Build history of the part. All positions in model axes, mm. Face numbers are marked on the shaded views. A direction names the side the tool comes from. Give positions to 0.01 mm unless a question says otherwise; leave off trailing zeros. Order: outer loops, then holes, each group sorted by start corner. A loop starts at its lowest first (then second) coordinate and runs counter-clockwise, first axis right, second up. Notation, with made-up numbers: (-19.75, -6) -> (-13.75, -6) arc R21 cw to (-13.75, 1) -> close; hole circle Ø1 at (88, 80.5). An arc over 180 degrees is marked (long way). Use a Markdown table: item, result. Add a question column.
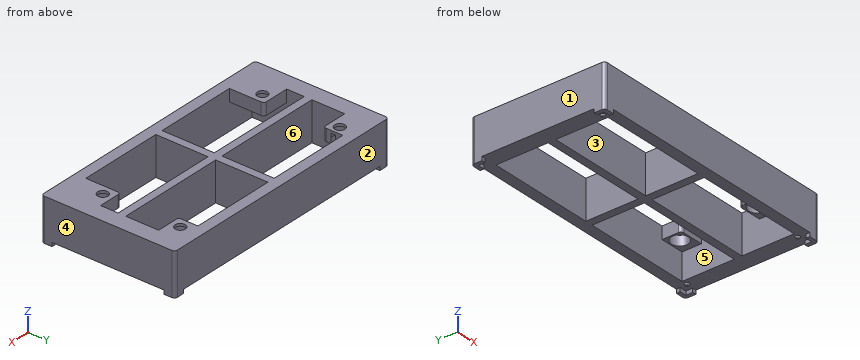
```python
from build123d import *

# Parameters (mm, degrees)
SKETCH1_W                                        = 170.1
SKETCH1_H                                        = 87.55
SKETCH1_W_2                                      = 148.1
SKETCH1_H_2                                      = 73.55
SKETCH1_W_3                                      = 71.55
SKETCH1_H_3                                      = 5
SKETCH1_W_4                                      = 5
SKETCH1_H_4                                      = 34.275
BOSS_EXTRUDE1_DEPTH                              = 25.4
SKETCH2_W                                        = 2.5
SKETCH2_H                                        = 4.5
SKETCH2_W_2                                      = 4.501529918
SKETCH2_H_2                                      = 2.5
SKETCH2_W_3                                      = 4.5
BOSS_EXTRUDE2_DEPTH                              = 2.5
SKETCH3_R                                        = 1.5
BOSS_EXTRUDE3_DEPTH                              = 1
BOSS_EXTRUDE4_DEPTH                              = 8
CBORE_FOR_1_4_SOCKET_HEAD_CAP_SCREW1_D           = 6.7564
CBORE_FOR_1_4_SOCKET_HEAD_CAP_SCREW1_CBORE_D     = 11.1125
CBORE_FOR_1_4_SOCKET_HEAD_CAP_SCREW1_CBORE_DEPTH = 6.35
FILLET1_R                                        = 1
FILLET2_R                                        = 2


with BuildPart() as part:
    # Sketch1 → Boss-Extrude1 (new body)
    # profile 1 of 6: a face of its own
    with BuildSketch(Plane.XY):
        with Locations((-57.284342841, -127.375162174)):
            Rectangle(SKETCH1_W, SKETCH1_H)
        with Locations((-57.284342841, -127.375162174)):
            Rectangle(SKETCH1_W_2, SKETCH1_H_2, mode=Mode.SUBTRACT)
    # profile 2 of 6: a face of its own
    with BuildSketch(Plane.XY):
        with Locations((-95.559342841, -127.375162174)):
            Rectangle(SKETCH1_W_3, SKETCH1_H_3)
    # profile 3 of 6: a face of its own
    with BuildSketch(Plane.XY):
        with Locations((-57.284342841, -107.737662174)):
            Rectangle(SKETCH1_W_4, SKETCH1_H_4)
    # profile 4 of 6: a face of its own
    with BuildSketch(Plane.XY):
        with Locations((-19.009342841, -127.375162174)):
            Rectangle(SKETCH1_W_3, SKETCH1_H_3)
    # profile 5 of 6: a face of its own
    with BuildSketch(Plane.XY):
        with Locations((-57.284342841, -147.012662174)):
            Rectangle(SKETCH1_W_4, SKETCH1_H_4)
    # profile 6 of 6: a face of its own
    with BuildSketch(Plane.XY):
        with Locations((-57.284342841, -127.375162174)):
            Rectangle(SKETCH1_W_4, SKETCH1_H_3)
    extrude(amount=BOSS_EXTRUDE1_DEPTH)

    # Sketch2 → Boss-Extrude2 (add)
    with BuildSketch(Plane(origin=(0, 0, 0), x_dir=(-1, 0, 0), z_dir=(0, 0, -1))):
        Polygon((135.334342841, -168.650162174), (135.334342841, -171.150162174), (142.334342841, -171.150162174), (142.334342841, -168.650162174), (139.834342841, -168.650162174), align=None)
        with Locations((141.084342841, -166.400162174)):
            Rectangle(SKETCH2_W, SKETCH2_H)
        Polygon((139.834342841, -90.600162174), (142.334342841, -90.600162174), (142.334342841, -83.600162174), (139.834342841, -83.600162174), (139.834342841, -86.100162174), align=None)
        with Locations((137.583577882, -84.850162174)):
            Rectangle(SKETCH2_W_2, SKETCH2_H_2)
        Polygon((-27.765657159, -83.600162174), (-27.765657159, -90.600162174), (-25.265657159, -90.600162174), (-25.265657159, -86.100162174), (-25.265657159, -83.600162174), align=None)
        with Locations((-23.015657159, -84.850162174)):
            Rectangle(SKETCH2_W_3, SKETCH2_H_2)
        Polygon((-27.765657159, -164.150162174), (-27.765657159, -171.150162174), (-25.265657159, -171.150162174), (-25.265657159, -168.650162174), (-25.265657159, -164.150162174), align=None)
        with Locations((-23.015657159, -169.900162174)):
            Rectangle(SKETCH2_W_3, SKETCH2_H_2)
    extrude(amount=BOSS_EXTRUDE2_DEPTH)

    # Sketch3 → Boss-Extrude3 (add)
    with BuildSketch(Plane(origin=(0, 0, 0), x_dir=(-1, 0, 0), z_dir=(0, 0, -1))):
        with Locations(Location((-20.265657159, -163.650162174, 0), (0, 0, 180))):
            Circle(SKETCH3_R)
        with Locations(Location((-20.265657159, -91.100162174, 0), (0, 0, 180))):
            Circle(SKETCH3_R)
        with Locations(Location((134.834342841, -163.650162174, 0), (0, 0, 180))):
            Circle(SKETCH3_R)
    extrude(amount=BOSS_EXTRUDE3_DEPTH)

    # Sketch4 → Boss-Extrude4 (add)
    with BuildSketch(Plane.XY.offset(25.4)):
        with BuildLine():
            Line((16.765657159, -90.600162174), (0.915657159, -90.600162174))
            Line((0.915657159, -90.600162174), (0.915657159, -101.300162174))
            ThreePointArc((0.915657159, -101.300162174), (1.501443597, -102.714375736), (2.915657159, -103.300162174))
            Line((2.915657159, -103.300162174), (16.765657159, -103.300162174))
            Line((16.765657159, -103.300162174), (16.765657159, -90.600162174))
        make_face()
        with BuildLine():
            Line((-131.334342841, -164.150162174), (-113.384342841, -164.150162174))
            Line((-113.384342841, -164.150162174), (-113.384342841, -143.400162174))
            ThreePointArc((-113.384342841, -143.400162174), (-113.970129278, -141.985948611), (-115.384342841, -141.400162174))
            Line((-115.384342841, -141.400162174), (-131.334342841, -141.400162174))
            Line((-131.334342841, -141.400162174), (-131.334342841, -164.150162174))
        make_face()
        with BuildLine():
            Line((-131.334342841, -90.600162174), (-114.384342841, -90.600162174))
            Line((-114.384342841, -90.600162174), (-114.384342841, -101.300162174))
            ThreePointArc((-114.384342841, -101.300162174), (-114.970129278, -102.714375736), (-116.384342841, -103.300162174))
            Line((-116.384342841, -103.300162174), (-131.334342841, -103.300162174))
            Line((-131.334342841, -103.300162174), (-131.334342841, -90.600162174))
        make_face()
        with BuildLine():
            Line((16.765657159, -141.400162174), (2.915657159, -141.400162174))
            ThreePointArc((2.915657159, -141.400162174), (1.501443597, -141.985948611), (0.915657159, -143.400162174))
            Line((0.915657159, -143.400162174), (0.915657159, -164.150162174))
            Line((0.915657159, -164.150162174), (16.765657159, -164.150162174))
            Line((16.765657159, -164.150162174), (16.765657159, -141.400162174))
        make_face()
    extrude(amount=-BOSS_EXTRUDE4_DEPTH)

    # CBORE for 1/4 Socket Head Cap Screw1 (through all)
    with Locations(Plane(origin=(0, 0, 17.4), x_dir=(-1, 0, 0), z_dir=(0, 0, -1))):
        with Locations((-7.265657159, -147.750162174), (-7.265657159, -96.950162174), (119.734342841, -96.950162174), (119.734342841, -147.750162174)):
            CounterBoreHole(CBORE_FOR_1_4_SOCKET_HEAD_CAP_SCREW1_D / 2, CBORE_FOR_1_4_SOCKET_HEAD_CAP_SCREW1_CBORE_D / 2, CBORE_FOR_1_4_SOCKET_HEAD_CAP_SCREW1_CBORE_DEPTH)

    # Fillet1
    fillet1_edges = [part.edges().sort_by_distance(p)[0] for p in [
        (18.765657159, -163.650162174, -1),
        (18.765657159, -91.100162174, -1),
        (-136.334342841, -163.650162174, -1),
    ]]
    fillet(fillet1_edges, radius=FILLET1_R - 0.0001)  # a hair under: the kernel refuses the full size

    # Fillet2
    fillet2_edges = [part.edges().sort_by_distance(p)[0] for p in [
        (27.765657159, -83.600162174, 11.45),
        (27.765657159, -171.150162174, 11.45),
        (-142.334342841, -171.150162174, 11.45),
        (-142.334342841, -83.600162174, 11.45),
    ]]
    fillet(fillet2_edges, radius=FILLET2_R)


solid = part.part
```
(1) Band-saw the part on B-B on x = -88. Give the cut face in (y, z), plus the area to 3 significant figures.
(2) Wall check: probe 1 along Y at (x, z) = (-85, 6.5); probe 2 along X at (y, z) = (-100, 9); probe 3 along X at (y, z) = (-158, 20.75). Give the ranges that are in metal, low to high.
(3) Band-saw the part on D-D on y = -156. Give the cut face in (x, z).
(4) Mould opens along Y. For the marked faces 1, 2 and 3 say: released by +Y, released by -Y, zero draft, split by the parting line, or undercut.
(5) Tool access for the marked faces 4, 5 and 6: list every direction of +Z, -Z, +X, -X, +Y, -Y with a clear straight run to the whole face (end or side of a thin tool).
(6) Band-saw the part on C-C on z = 5.75. Give the cut face in (x, y), plus the area to 3 significant figures.
(7) Pin check, flat tips, straight feed: pin 1 Ø12.5 at (x, y) = (8, -154) entering from -Z; pin 2 Ø5.5 at (x, y) = (-121.5, -96) entering from -Z. Stop position of each tip, or through.
(8) Band-saw the part on A-A on y = -123. Give the cut face in (x, z).
Response:
| question | item | result |
|---|---|---|
| 1 | outline | (-171.15, 0) -> (-164.15, 0) -> (-164.15, 25.4) -> (-171.15, 25.4) -> close; (-129.88, 0) -> (-124.88, 0) -> (-124.88, 25.4) -> (-129.88, 25.4) -> close; (-90.6, 0) -> (-83.6, 0) -> (-83.6, 25.4) -> (-90.6, 25.4) -> close |
| 1 | area | 483 mm² |
| 2 | probe 1 | y = -171.15 to -164.15, -129.88 to -124.88, -90.6 to -83.6 |
| 2 | probe 2 | x = -142.33 to -131.33, -59.78 to -54.78, 16.77 to 27.77 |
| 2 | probe 3 | x = -142.33 to -113.38, -59.78 to -54.78, 0.92 to 27.77 |
| 3 | outline | (-142.33, 0) -> (-131.33, 0) -> (-131.33, 17.4) -> (-113.38, 17.4) -> (-113.38, 25.4) -> (-142.33, 25.4) -> close; (-59.78, 0) -> (-54.78, 0) -> (-54.78, 25.4) -> (-59.78, 25.4) -> close; (0.92, 17.4) -> (16.77, 17.4) -> (16.77, 0) -> (27.77, 0) -> (27.77, 25.4) -> (0.92, 25.4) -> close |
| 4 | face 1 | zero draft |
| 4 | face 2 | released by +Y |
| 4 | face 3 | undercut |
| 5 | face 4 | +Z, -Z, +X, +Y, -Y |
| 5 | face 5 | -Z |
| 5 | face 6 | +Z, -Z |
| 6 | outline | (-142.33, -169.15) arc R2 ccw to (-140.33, -171.15) -> (25.77, -171.15) arc R2 ccw to (27.77, -169.15) -> (27.77, -85.6) arc R2 ccw to (25.77, -83.6) -> (-140.33, -83.6) arc R2 ccw to (-142.33, -85.6) -> close; hole (-131.33, -164.15) -> (-59.78, -164.15) -> (-59.78, -129.88) -> (-131.33, -129.88) -> close; hole (-131.33, -124.88) -> (-59.78, -124.88) -> (-59.78, -90.6) -> (-131.33, -90.6) -> close; hole (-54.78, -164.15) -> (16.77, -164.15) -> (16.77, -129.88) -> (-54.78, -129.88) -> close; hole (-54.78, -124.88) -> (16.77, -124.88) -> (16.77, -90.6) -> (-54.78, -90.6) -> close |
| 6 | area | 5,080 mm² |
| 7 | pin 1 | stops at z = 17.4 |
| 7 | pin 2 | stops at z = 23.75 |
| 8 | outline | (-142.33, 0) -> (-131.33, 0) -> (-131.33, 25.4) -> (-142.33, 25.4) -> close; (-59.78, 0) -> (-54.78, 0) -> (-54.78, 25.4) -> (-59.78, 25.4) -> close; (16.77, 0) -> (27.77, 0) -> (27.77, 25.4) -> (16.77, 25.4) -> close |
